Build history of the part. All positions in model axes, mm. A direction names the side the tool comes from. Round coordinates to 2 decimals unless told otherwise and drop trailing zeros. Write each loop counter-clockwise with the first axis right and the second up, starting at its lowest first coordinate (ties: lowest second). Pieces come first, ordered by that corner, then holes.
from build123d import *

# Parameters (mm, degrees)
SKETCH1_W               = 111.013561953
SKETCH1_H               = 10
BOSS_EXTRUDE3_DEPTH     = 1.5875
CUT_EXTRUDE1_DEPTH      = 114.026682648
CUT_EXTRUDE1_DEPTH_BACK = 114.026682648
SKETCH2_R               = 6.5
SKETCH3_W               = 25.483030165
SKETCH3_H               = 20
BOSS_EXTRUDE4_DEPTH     = 10


with BuildPart() as part:
    # Sketch1 → Boss-Extrude3 (new, symmetric)
    with BuildSketch(Plane.XY):
        with Locations((-57.031880671, 5)):
            Rectangle(SKETCH1_W, SKETCH1_H)
        with Locations((-57.031880671, -5)):
            Rectangle(SKETCH1_W, SKETCH1_H)
    extrude(amount=BOSS_EXTRUDE3_DEPTH, both=True)

    # Sketch2 → Cut-Extrude1 (cut, two sides: drawn at the far end of the back side and taken through both)
    with BuildSketch(Plane.XY.offset(1.5875).offset(-CUT_EXTRUDE1_DEPTH_BACK)):
        with Locations((-50.538661647, 0)):
            Circle(SKETCH2_R)
    extrude(amount=CUT_EXTRUDE1_DEPTH + CUT_EXTRUDE1_DEPTH_BACK, mode=Mode.SUBTRACT)

    # Sketch3 → Boss-Extrude4 (add)
    with BuildSketch(Plane.XY.offset(1.5875)):
        with Locations((-99.797146565, 0)):
            Rectangle(SKETCH3_W, SKETCH3_H)
    extrude(amount=BOSS_EXTRUDE4_DEPTH)


solid = part.part
1) Which spindle directions (+Z, -Z, +X, -X, +Y, -Y) get a long thin tool onto all of the face, cutting with end or side? Do faces 5 (the flat face through (-45, 5, 1.588)), 6 (the flat face through (-82, -10, 1)). Say none if no direction does.
Results:
face 5: +Z, +X, +Y, -Y
face 6: +Z, -Z, +X, -X, -Y
2) Wall check: L1, parallel to X at y = 0, z = -0.9; L2, parallel to Z at x = -72.5, y = -9; L3, parallel to X at y = -8.25, z = 4. Give the ranges that are in metal, low to high.
Results:
L1: x = -112.54 to -57.04, -44.04 to -1.53
L2: z = -1.59 to 1.59
L3: x = -112.54 to -87.06
3) Slice it at A-A (y = 0). Write the cut outline in (x, z), plus the area to 3 significant figures.
Results:
outline: (-112.54, -1.59) - (-57.04, -1.59) - (-57.04, 1.59) - (-87.06, 1.59) - (-87.06, 11.59) - (-112.54, 11.59) - close; (-44.04, -1.59) - (-1.53, -1.59) - (-1.53, 1.59) - (-44.04, 1.59) - close
area: 566 mm2
4) Mould opens along X. For faces 1 (the flat face through (-1.525, 0, 0)), 2 (the flat face through (-112.539, 0, 5)), 3 (the flat face through (-58, 0, -1.588)), 4 (the cylindrical face through (-44.34, 1.95, -0.02)) say: released by +X, released by -X, zero draft, split by the parting line, or undercut.
Results:
face 1: released by +X
face 2: released by -X
face 3: zero draft
face 4: undercut
5) Slice it at D-D (z = 4.5). Write the cut outline in (x, y), plus the area to 3 significant figures.
Results:
outline: (-112.54, -10) - (-87.06, -10) - (-87.06, 10) - (-112.54, 10) - close
area: 510 mm2
6) Pin check, flat tips, straight feed: pin 1 Ø4 at (x, y) = (-20.5, -7.5) entering from +Z; pin 2 Ø1 at (y, z) = (7.5, 6.5) entering from +X. Stop position of each tip, or through.
Results:
pin 1: stops at z = 1.59
pin 2: stops at x = -87.06
7) Slice it at B-B (x = -55). Write the cut outline in (y, z).
Results:
outline: (-10, -1.59) - (-4.73, -1.59) - (-4.73, 1.59) - (-10, 1.59) - close; (4.73, -1.59) - (10, -1.59) - (10, 1.59) - (4.73, 1.59) - close
8) Slice it at C-C (y = 8.25). Write the cut outline in (x, z), plus the area to 3 significant figures.
Results:
outline: (-112.54, -1.59) - (-1.53, -1.59) - (-1.53, 1.59) - (-87.06, 1.59) - (-87.06, 11.59) - (-112.54, 11.59) - close
area: 607 mm2
